Read the model definition and answer for the solid it produces. Units are mm, in the model's axes. A direction names the side the tool comes from. Round coordinates to 2 decimals unless told otherwise and drop trailing zeros. Order: outer loops, then holes, each group sorted by start corner. A loop starts at its lowest first (then second) coordinate and runs counter-clockwise, first axis right, second up. Notation, with made-up numbers: (-30, 13.25) -> (-16, 13.25) arc R28 cw to (-16, 36.25) -> close; hole circle Ø4 at (14, -13). An arc over 180 degrees is marked (long way). Answer as a JSON object with one key per item and string values. Group by question number.
Item 1: For faces 4 (the flat face through (1168.4, -253, -63)), 5 (the flat face through (1193.8, -253, -63)), 6 (the flat face through (-64, -127, -1143)), determine the directions among +Z, -Z, +X, -X, +Y, -Y from which every point of the face is accessible in a straight line to the end or side of a thin tool.
Item 2: Section D-D, the plane x = 966.5 is taken. Write down the section's boundary in (y, z), plus the area to 3 significant figures.
Item 3: Section C-C, the plane z = -618 is taken. Write down the section's boundary in (x, y).
Item 4: Section A-A, the plane y = 101.6 is taken. Write down the section's boundary in (x, z).
Item 5: The mould has two halves that part along Z. Classify faces 1 (the flat face through (1156, -253, -1168.4)), 2 (the flat face through (-64, -127, -76.2)), 3 (the flat face through (-63, -101, -1092.2)): pulls with the +Z half, pulls with the -Z half, needs draft (parallel to the pull), parting line crosses it, or undercut.
Item 6: Given P1, Ø12.5, axis at x = 1104, y = -273.5, coming from the +Z side; P2, Ø23, axis at y = -263, z = -98.5, coming from the -X side; P3, Ø4, axis at y = 61, z = -1000.5, coming from the -X side, each flat-ended and moving along its own axis, determine where each tip first touches the part or whether it passes through.
Item 7: Consider probe 1 along X at (y, z) = (101, -81); probe 2 along Y at (x, z) = (452, -793); probe 3 along Y at (x, z) = (1130, -1110). Determine where each line is inside the solid, lowest interval first. Write a range as from..to.
Item 8: Section B-B, the plane x = -63.5 is taken. Write down the section's boundary in (y, z), plus the area to 3 significant figures.
from build123d import *

# Parameters (mm, degrees)
BOSS_EXTRUDE1_DEPTH = 203.2
SKETCH2_W           = 1016
SKETCH2_H           = 1016
CUT_EXTRUDE1_DEPTH  = 50.8
SKETCH3_W           = 1016
SKETCH3_H           = 1016
CUT_EXTRUDE2_DEPTH  = 50.8
SKETCH4_W           = 1016
SKETCH4_H           = 101.6
CUT_EXTRUDE3_DEPTH  = 50.8
SKETCH5_W           = 1016
SKETCH5_H           = 101.6
CUT_EXTRUDE4_DEPTH  = 50.8
SKETCH6_R           = 50.8
CUT_EXTRUDE5_DEPTH  = 1270
SKETCH7_R           = 50.8
CUT_EXTRUDE6_DEPTH  = 1270
SKETCH8_W           = 1219.2
SKETCH8_H           = 101.6
BOSS_EXTRUDE2_DEPTH = 101.6
SKETCH9_W           = 1219.2
SKETCH9_H           = 1219.2
BOSS_EXTRUDE4_DEPTH = 101.6
SKETCH10_W          = 25.4
SKETCH10_H          = 76.2
SKETCH10_W_2        = 76.2
SKETCH10_H_2        = 25.4
BOSS_EXTRUDE5_DEPTH = 101.6
SKETCH12_R          = 25.4
CUT_EXTRUDE7_DEPTH  = 203.2
SKETCH13_R          = 25.4
CUT_EXTRUDE8_DEPTH  = 203.2
SKETCH14_R          = 25.4
CUT_EXTRUDE9_DEPTH  = 203.2
SKETCH15_R          = 25.4
CUT_EXTRUDE10_DEPTH = 203.2
SKETCH16_W          = 1016
SKETCH16_H          = 50.8
BOSS_EXTRUDE6_DEPTH = 1219.2
BOSS_EXTRUDE7_DEPTH = 127
SKETCH18_R          = 25.4
BOSS_EXTRUDE8_DEPTH = 50.8
BOSS_EXTRUDE9_START = 50.8
SKETCH19_R          = 25.4
BOSS_EXTRUDE9_DEPTH = 50.8


with BuildPart() as part:
    # Sketch1 → Boss-Extrude1 (new body)
    with BuildSketch(Plane(origin=(0, 0, 0), x_dir=(1, 0, 0), z_dir=(0, 1, 0))):
        Polygon((0, 0), (1219.2, 0), (1219.2, 101.6), (1117.6, 101.6), (1117.6, 1117.6), (1219.2, 1117.6), (1219.2, 1219.2), (0, 1219.2), (0, 1117.6), (101.6, 1117.6), (101.6, 101.6), (0, 101.6), align=None)
    extrude(amount=BOSS_EXTRUDE1_DEPTH)

    # Sketch2 → Cut-Extrude1 (cut)
    with BuildSketch(Plane(origin=(0, 203.2, 0), x_dir=(1, 0, 0), z_dir=(0, 1, 0))):
        with Locations((609.6, 609.6)):
            Rectangle(SKETCH2_W, SKETCH2_H)
    extrude(amount=-CUT_EXTRUDE1_DEPTH, mode=Mode.SUBTRACT)

    # Sketch3 → Cut-Extrude2 (cut)
    with BuildSketch(Plane(origin=(0, 0, 0), x_dir=(-1, 0, 0), z_dir=(0, -1, 0))):
        with Locations((-609.6, 609.6)):
            Rectangle(SKETCH3_W, SKETCH3_H)
    extrude(amount=-CUT_EXTRUDE2_DEPTH, mode=Mode.SUBTRACT)

    # Sketch4 → Cut-Extrude3 (cut)
    with BuildSketch(Plane(origin=(1117.6, 0, 0), x_dir=(0, 0, -1), z_dir=(1, 0, 0))):
        with Locations((609.6, 101.6)):
            Rectangle(SKETCH4_W, SKETCH4_H)
    extrude(amount=-CUT_EXTRUDE3_DEPTH, mode=Mode.SUBTRACT)

    # Sketch5 → Cut-Extrude4 (cut)
    with BuildSketch(Plane.ZY.offset(-101.6)):
        with Locations((-609.6, 101.6)):
            Rectangle(SKETCH5_W, SKETCH5_H)
    extrude(amount=-CUT_EXTRUDE4_DEPTH, mode=Mode.SUBTRACT)

    # Sketch6 → Cut-Extrude5 (cut)
    with BuildSketch(Plane.XY):
        with Locations((1143, 101.6)):
            Circle(SKETCH6_R)
    extrude(amount=-CUT_EXTRUDE5_DEPTH, mode=Mode.SUBTRACT)

    # Sketch7 → Cut-Extrude6 (cut)
    with BuildSketch(Plane(origin=(0, 0, -1219.2), x_dir=(-1, 0, 0), z_dir=(0, 0, -1))):
        with Locations((-76.2, 101.6)):
            Circle(SKETCH7_R)
    extrude(amount=-CUT_EXTRUDE6_DEPTH, mode=Mode.SUBTRACT)

    # Sketch8 → Boss-Extrude2 (add)
    with BuildSketch(Plane(origin=(0, 0, 0), x_dir=(-1, 0, 0), z_dir=(0, -1, 0))):
        with Locations((-609.6, 50.8)):
            Rectangle(SKETCH8_W, SKETCH8_H)
        with Locations((-609.6, 1168.4)):
            Rectangle(SKETCH8_W, SKETCH8_H)
    extrude(amount=BOSS_EXTRUDE2_DEPTH)

    # Sketch9 → Boss-Extrude4 (add)
    with BuildSketch(Plane(origin=(0, -101.6, 0), x_dir=(-1, 0, 0), z_dir=(0, -1, 0))):
        with Locations((-609.6, 609.6)):
            Rectangle(SKETCH9_W, SKETCH9_H)
    extrude(amount=BOSS_EXTRUDE4_DEPTH)

    # Sketch10 → Boss-Extrude5 (add)
    with BuildSketch(Plane(origin=(0, -203.2, 0), x_dir=(-1, 0, 0), z_dir=(0, -1, 0))):
        with Locations((-1104.9, 88.9)):
            Rectangle(SKETCH10_W, SKETCH10_H)
        with Locations((-1181.1, 88.9)):
            Rectangle(SKETCH10_W, SKETCH10_H)
        with Locations((-88.9, 114.3)):
            Rectangle(SKETCH10_W_2, SKETCH10_H_2)
        with Locations((-88.9, 35.337450191)):
            Rectangle(SKETCH10_W_2, SKETCH10_H_2)
        with Locations((-1130.3, 1104.9)):
            Rectangle(SKETCH10_W_2, SKETCH10_H_2)
        with Locations((-1130.3, 1181.1)):
            Rectangle(SKETCH10_W_2, SKETCH10_H_2)
        with Locations((-38.1, 1130.3)):
            Rectangle(SKETCH10_W, SKETCH10_H)
        with Locations((-114.3, 1130.3)):
            Rectangle(SKETCH10_W, SKETCH10_H)
    extrude(amount=BOSS_EXTRUDE5_DEPTH)

    # Sketch12 → Cut-Extrude7 (cut)
    with BuildSketch(Plane(origin=(1193.8, 0, 0), x_dir=(0, 0, -1), z_dir=(1, 0, 0))):
        with Locations((88.9, -254)):
            Circle(SKETCH12_R)
    extrude(amount=-CUT_EXTRUDE7_DEPTH, mode=Mode.SUBTRACT)

    # Sketch13 → Cut-Extrude8 (cut)
    with BuildSketch(Plane(origin=(0, 0, -1193.8), x_dir=(-1, 0, 0), z_dir=(0, 0, -1))):
        with Locations((-1130.3, -254)):
            Circle(SKETCH13_R)
    extrude(amount=-CUT_EXTRUDE8_DEPTH, mode=Mode.SUBTRACT)

    # Sketch14 → Cut-Extrude9 (cut)
    with BuildSketch(Plane.ZY.offset(-25.4)):
        with Locations(Location((-1130.3, -254, 0), (0, 0, 180))):
            Circle(SKETCH14_R)
    extrude(amount=-CUT_EXTRUDE9_DEPTH, mode=Mode.SUBTRACT)

    # Sketch15 → Cut-Extrude10 (cut)
    with BuildSketch(Plane.XY.offset(-22.637450191)):
        with Locations((88.9, -254)):
            Circle(SKETCH15_R)
    extrude(amount=-CUT_EXTRUDE10_DEPTH, mode=Mode.SUBTRACT)

    # Sketch16 → Boss-Extrude6 (add)
    with BuildSketch(Plane.ZY):
        with Locations((-609.6, -76.2)):
            Rectangle(SKETCH16_W, SKETCH16_H)
    extrude(amount=-BOSS_EXTRUDE6_DEPTH)

    # Sketch17 → Boss-Extrude7 (add)
    with BuildSketch(Plane.ZY):
        Polygon((-1092.2, -165.1), (-1041.4, -165.1), (-1041.4, -127), (-1041.4, -88.9), (-1092.2, -88.9), align=None)
        Polygon((-177.8, -127), (-177.8, -88.9), (-127, -88.9), (-127, -165.1), (-177.8, -165.1), align=None)
    extrude(amount=BOSS_EXTRUDE7_DEPTH)

    # Sketch18 → Boss-Extrude8 (add)
    with BuildSketch(Plane(origin=(0, 0, -1092.2), x_dir=(-1, 0, 0), z_dir=(0, 0, -1))):
        with Locations(Location((63.5, -127, 0), (0, 0, 180))):
            Circle(SKETCH18_R)
    extrude(amount=BOSS_EXTRUDE8_DEPTH)

    # Sketch19 → Boss-Extrude9 (add)
    with BuildSketch(Plane.XY.offset(-127).offset(BOSS_EXTRUDE9_START)):
        with Locations((-63.5, -127)):
            Circle(SKETCH19_R)
    extrude(amount=-BOSS_EXTRUDE9_DEPTH)


solid = part.part
Values found:
{
 "1": {"face 4": "+Z, -Y", "face 5": "+Z, -Z, +X, -Y", "face 6": "-Z, -X, +Y, -Y"},
 "2": {"outline": "(-203.2, -1219.2) -> (203.2, -1219.2) -> (203.2, -1117.6) -> (152.4, -1117.6) -> (152.4, -101.6) -> (203.2, -101.6) -> (203.2, 0) -> (-203.2, 0) -> close; hole (-50.8, -1117.6) -> (50.8, -1117.6) -> (50.8, -101.6) -> (-50.8, -101.6) -> close", "area": "341,000 mm2"},
 "3": {"outline": "(0, -203.2) -> (1219.2, -203.2) -> (1219.2, -50.8) -> (0, -50.8) -> close; (152.4, 50.8) -> (1066.8, 50.8) -> (1066.8, 152.4) -> (152.4, 152.4) -> close"},
 "4": {"outline": "(0, -1219.2) -> (25.4, -1219.2) -> (25.4, -1117.6) -> (0, -1117.6) -> close; (0, -101.6) -> (25.4, -101.6) -> (25.4, 0) -> (0, 0) -> close; (127, -1219.2) -> (1092.2, -1219.2) -> (1092.2, -1117.6) -> (1066.8, -1117.6) -> (1066.8, -101.6) -> (1092.2, -101.6) -> (1092.2, 0) -> (127, 0) -> (127, -101.6) -> (152.4, -101.6) -> (152.4, -1117.6) -> (127, -1117.6) -> close; (1193.8, -1219.2) -> (1219.2, -1219.2) -> (1219.2, -1117.6) -> (1193.8, -1117.6) -> close; (1193.8, -101.6) -> (1219.2, -101.6) -> (1219.2, 0) -> (1193.8, 0) -> close"},
 "5": {"face 1": "undercut", "face 2": "pulls with the +Z half", "face 3": "pulls with the -Z half"},
 "6": {"P1": "z = -50.8", "P2": "x = 50.8", "P3": "x = 152.4"},
 "7": {"probe 1": "0..25.4, 127..1092.2, 1193.8..1219.2", "probe 2": "-203.2..-50.8, 50.8..152.4", "probe 3": "-304.8..-279.4, -228.6..-50.8"},
 "8": {"outline": "(-165.1, -1092.2) -> (-152.4, -1092.2) -> (-152.4, -1143) -> (-101.6, -1143) -> (-101.6, -1092.2) -> (-88.9, -1092.2) -> (-88.9, -1041.4) -> (-165.1, -1041.4) -> close; (-165.1, -177.8) -> (-88.9, -177.8) -> (-88.9, -127) -> (-101.6, -127) -> (-101.6, -76.2) -> (-152.4, -76.2) -> (-152.4, -127) -> (-165.1, -127) -> close", "area": "12,900 mm2"}
}
